Autodesk Fusion 360 part; units mm, degrees
sketch "Sketch1" plane through (0, 0, 0) normal (0, 0, 1) x (1, 0, 0)
  line L0 (0, 0) -> (15, 0)
  line L1 (15, 0) -> (15, 15)
  line L2 (15, 15) -> (0, 15)
  line L3 (0, 15) -> (0, 0)
  dimension "d1" = 15
  dimension "d2" = 15
extrude "Extrude1" add sketch "Sketch1" along normal blind 35
extrude "Extrude2" add 1 faces at (5, 10, 35) along direction (0, 0, 1) blind 3
sketch "Sketch2" plane through (15, 0, 0) normal (1, 0, 0) x (0, 1, 0)
  line L0 (0, 0) -> (15, 0)
  line L1 (15, 0) -> (15, 38)
  line L2 (15, 38) -> (0, 38)
  line L3 (0, 38) -> (0, 0)
  line L4 (0, 38) -> (15, 38)
  line L5 (15, 38) -> (15, 35.5)
  line L6 (15, 35.5) -> (0, 35.5)
  line L7 (0, 35.5) -> (0, 38)
  line L8 (0, 35.5) -> (15, 35.5)
  line L9 (15, 35.5) -> (15, 30.5)
  line L10 (15, 30.5) -> (0, 30.5)
  line L11 (0, 30.5) -> (0, 35.5)
  line L12 (0, 30.5) -> (15, 30.5)
  line L13 (15, 30.5) -> (15, 15.5)
  line L14 (15, 15.5) -> (0, 15.5)
  line L15 (0, 15.5) -> (0, 30.5)
  line L16 (0, 30.5) -> (15, 15.5)
  line L17 (15, 30.5) -> (0, 15.5)
  circle A0 centre (7.5, 23) radius 3.5
  dimension "d7" = 2.5
  dimension "d8" = 5
  dimension "d9" = 15
  dimension "d10" = 7
extrude "Extrude3" cut sketch "Sketch2" against normal blind 45 contours L16 L17 A0 | L16 L17 A0 | L16 L17 A0 | L16 L17 A0
sketch "Sketch3" plane through (0, 0, 0) normal (0, -1, 0) x (1, 0, 0)
  line L0 (0, 0) -> (15, 0)
  line L1 (15, 0) -> (15, 38)
  line L2 (15, 38) -> (0, 38)
  line L3 (0, 38) -> (0, 0)
  line L4 (0, 0) -> (15, 0)
  line L5 (15, 0) -> (15, 15)
  line L6 (15, 15) -> (0, 15)
  line L7 (0, 15) -> (0, 0)
  line L8 (0, 15) -> (15, 0)
  line L9 (15, 15) -> (0, 0)
  circle A0 centre (7.5, 7.5) radius 2.5
  dimension "d13" = 15
  dimension "d14" = 15
  dimension "d15" = 5
extrude "Extrude4" cut sketch "Sketch3" against normal blind 45 contours L8 L9 A0 | L8 L9 A0 | L8 L9 A0 | L8 L9 A0
The model under review builds one solid part; all positions refer to its coordinate system, in mm. Give positions to 0.01 mm unless a question says otherwise; leave off trailing zeros. Order: outer loops, then holes, each group sorted by start corner. A loop starts at its lowest first (then second) coordinate and runs counter-clockwise, first axis right, second up. Notation, with made-up numbers: (77, -33.5) -> (136, -33.5) arc R22 cw to (136, -11.5) -> close; hole circle Ø3 at (5.5, -12). An arc over 180 degrees is marked (long way). Write item = value, one per line. Start each with the question number.
(1) For L1, parallel to Y at x = 9.5, z = 23; L2, parallel to Z at x = 9.75, y = 7.5; L3, parallel to Z at x = 6.5, y = 7, list the stretches that pass through material, from the lowest coordinate up. Write a range as from..to.
(2) Take a section at A-A (x = 7.5). Write out the cut boundary in (y, z).
(3) Draft analysis for pull direction Z (two halves, no side actions). For faces 1 (the cylindrical face through (7.6, 7.04, 26.47)), 2 (the flat face through (7, 8, 0)), 3 (the flat face through (15, 7, 19)), state which applies: +Z half, -Z half, draft (parallel to the pull), parting line (faces both ways), or undercut.
(4) For pin 1 Ø4 at (x, y) = (13, 3.5) entering from -Z, flat-tipped, find the tip position at first contact; note if it passes through.
(5) Take a section at D-D (x = 13.25). Write out the cut boundary in (y, z).
(6) Take a section at C-C (z = 9.5). Write out the cut boundary in (x, y).
(7) Take a section at B-B (y = 7.5). Write out the cut boundary in (x, z).
Returned:
q1.L1 = 0..4, 11..15
q1.L2 = 0..6.41, 8.59..19.5, 26.5..38
q1.L3 = 0..5.21, 9.79..19.54, 26.46..38
q2.outline = (0, 0) -> (15, 0) -> (15, 5) -> (0, 5) -> close; (0, 10) -> (15, 10) -> (15, 38) -> (0, 38) -> close; hole circle Ø7 at (7.5, 23)
q3.face_1 = undercut
q3.face_2 = -Z half
q3.face_3 = draft
q4.pin_1 = 0
q5.outline = (0, 0) -> (15, 0) -> (15, 38) -> (0, 38) -> close; hole circle Ø7 at (7.5, 23)
q6.outline = (0, 0) -> (6, 0) -> (6, 15) -> (0, 15) -> close; (9, 0) -> (15, 0) -> (15, 15) -> (9, 15) -> close
q7.outline = (0, 0) -> (15, 0) -> (15, 19.5) -> (0, 19.5) -> close; (0, 26.5) -> (15, 26.5) -> (15, 38) -> (0, 38) -> close; hole circle Ø5 at (7.5, 7.5)
